Autodesk Inventor part; units mm, degrees
ref_plane "YZ Plane" through (0, 0, 0) normal (1, 0, 0) x (0, 1, 0)
ref_plane "XZ Plane" through (0, 0, 0) normal (0, 1, 0) x (-1, 0, 0)
ref_plane "XY Plane" through (0, 0, 0) normal (0, 0, 1) x (1, 0, 0)
sketch "スケッチ1" plane through (0, 0, 0) normal (1, 0, 0) x (0, 1, 0)
  line L0 (10, 0) -> (0, 0)
  line L1 (0, 0) -> (0, -15)
  line L2 (0, -15) -> (10, -15)
  line L3 (10, -15) -> (10, 0)
  line L4 (10, 0) -> (0, 0)
  line L5 (0, 0) -> (0, 6.0622)
  line L6 (0, 6.0622) -> (10, 6.0622)
  line L7 (10, 6.0622) -> (10, 0)
  line L8 (0, 6.0622) -> (3.5, 0)
  line L9 (3.5, 0) -> (29.4808, 15)
  line L10 (29.4808, 15) -> (25.9808, 21.0622)
  line L11 (25.9808, 21.0622) -> (0, 6.0622)
  arc A0 (29.4808, 15) -> (17.3205, 16.0622) centre (22.6419, 6.8452) ccw
  point P0 (10, 3.7528)
  dimension "d0" = 10
  dimension "d1" = 15
  dimension "d6" = 30
  dimension "d10" = 60
  dimension "d11" = 7
  dimension "d12" = 20
extrude "押し出し1" add sketch "スケッチ1" along normal blind 1.5 contours L3 L2 L1 L0 | L0 L9 L7 | L0 L5 L8 | L8 L6 L7 L9 | L7 L6 L11 A0 L9
fillet "フィレット2" radius 5 1 edges at (0.75, 10, 3.7528)
sketch "スケッチ2" plane through (1.5, 0, 0) normal (1, 0, 0) x (0, 0, -1)
  circle A0 centre (10, 5) radius 0.8
  circle A1 centre (5, 5) radius 0.8
  line L0 (15, 0) -> (15, 10)
  point P0 (0, 0)
  point P1 (15, 5)
  dimension "d14" = 1.6
  dimension "d15" = 1.6
  dimension "d16" = 5
  dimension "d17" = 5
extrude "押し出し2" cut sketch "スケッチ2" against normal through all
properties part number "claw2"
Geometry check sheet. Reference: the model listing, model coordinates, mm. A direction names the side the tool comes from. Coordinates: 2 decimals unless noted, no trailing zeros. Order: outer loops, then holes, each group sorted by start corner. A loop starts at its lowest first (then second) coordinate and runs counter-clockwise, first axis right, second up. Notation, with made-up numbers: (15, 62.25) -> (28, 62.25) arc R21 cw to (28, 96.25) -> close; hole circle Ø4 at (78, 63). An arc over 180 degrees is marked (long way). Use a Markdown table: item, result. Add a question column.
1. Cross-section at D-D (y = 8.25). Enter the section's corners in (x, z), and give its area (3 significant figures).
2. Cross-section at A-A (z = -10). Enter the section's corners in (x, y).
3. Cross-section at B-B (y = 5). Enter the section's corners in (x, z), and give its area (3 significant figures).
4. Material ranges on L1, parallel to Y at x = 0.3, z = -5; L2, parallel to Y at x = 0.65, z = -9; L3, parallel to Y at x = 0.55, z = 7, recorded low to high.
5. Cross-section at C-C (x = 0.6). Enter the section's corners in (y, z), and give its area (3 significant figures).
6. Mould release check, pull along Y, two halves, no side actions. Record for faces 1 (the face through (1, 5, -15)), 2 (the face through (0.74, 20.87, 10.03)), 3 (the face through (1, 0, -4)), 4 (the face through (0.76, 4.51, -9.37)): pulls with the +Y half, pulls with the -Y half, needs draft (parallel to the pull), parting line crosses it, or undercut.
7. Set-up check for faces 5 (the face through (1.5, 11, 5)), 6 (the face through (1, 10, -7)): record each of +Z, -Z, +X, -X, +Y, -Y from which the full face is reachable in a straight line by a thin tool's end or side.
Filled sheet:
| question | item | result |
|---|---|---|
| 1 | outline | (0, -15) -> (1.5, -15) -> (1.5, 10.83) -> (0, 10.83) -> close |
| 1 | area | 38.7 mm2 |
| 2 | outline | (0, 0) -> (1.5, 0) -> (1.5, 4.2) -> (0, 4.2) -> close; (0, 5.8) -> (1.5, 5.8) -> (1.5, 10) -> (0, 10) -> close |
| 3 | outline | (0, -15) -> (1.5, -15) -> (1.5, -10.8) -> (0, -10.8) -> close; (0, -9.2) -> (1.5, -9.2) -> (1.5, -5.8) -> (0, -5.8) -> close; (0, -4.2) -> (1.5, -4.2) -> (1.5, 8.95) -> (0, 8.95) -> close |
| 3 | area | 31.1 mm2 |
| 4 | L1 | 0 to 4.2, 5.8 to 10 |
| 4 | L2 | 0 to 10 |
| 4 | L3 | 1.62 to 15.62 |
| 5 | outline | (0, -15) -> (10, -15) -> (10, 0.87) arc R5 cw to (12.5, 5.2) -> (29.48, 15) arc R10.64 ccw to (17.32, 16.06) -> (0, 6.06) -> close; hole circle Ø1.6 at (5, -10); hole circle Ø1.6 at (5, -5) |
| 5 | area | 361 mm2 |
| 6 | face 1 | needs draft |
| 6 | face 2 | pulls with the +Y half |
| 6 | face 3 | pulls with the -Y half |
| 6 | face 4 | undercut |
| 7 | face 5 | +Z, -Z, +X, +Y, -Y |
| 7 | face 6 | -Z, +X, -X, +Y |
